Source: CAD feature listing. Evaluate the final solid. Frame: model axes, mm. Face numbers are marked on the shaded views. Give positions to 0.01 mm unless a question says otherwise; leave off trailing zeros. Write each loop counter-clockwise with the first axis right and the second up, starting at its lowest first coordinate (ties: lowest second). Pieces come first, ordered by that corner, then holes. Notation, with made-up numbers: (86, 58) -> (111, 58) arc R19 ccw to (111, 76) -> close; hole circle Ø5 at (85, 41.25). An arc over 180 degrees is marked (long way). Answer as a JSON object with one key per item and string values. Group by question number.
Item 1: Ray query, probe 1 along Z at (x, y) = (8.5, 18.5); probe 2 along X at (y, z) = (25, 232.5); probe 3 along Y at (x, z) = (-34, 32). Return the intervals inside material, ascending. Write a range as from..to.
Item 2: Section query A-A on y = 0. Return the cut outline in (x, z).
Item 3: Section query C-C on y = 13. Return the cut outline in (x, z).
Item 4: Section query D-D on z = 16.5. Return the cut outline in (x, y), plus the area to 3 significant figures.
Item 5: Section query B-B on x = 0. Return the cut outline in (y, z), plus the area to 3 significant figures.
Item 6: Pull-direction query (Y, two-part tool) for the marked faces 1, 2, 3 and 4; classes: pulls with the +Y half, pulls with the -Y half, needs draft (parallel to the pull), parting line crosses it, or undercut.
Item 7: First-contact query: pin 1 Ø10 at (x, z) = (30, 86.5) entering from -Y; pin 2 Ø5 at (y, z) = (-1, 162.5) entering from -X; pin 3 Ø3 at (x, z) = (-19, 105.5) entering from +Y. Flat tips, straight axial feed; report the tip coordinate or a pass-through.
from build123d import *

# Parameters (mm, degrees)
F0_R          = 50
F1_DEPTH      = 250
F2_W          = 50
F2_H          = 26.758289
F3_DEPTH      = 50
F3_DEPTH_BACK = 50


with BuildPart() as f1:
    # F0 (on Top) → F1 (new body)
    with BuildSketch(Plane.XY):
        Circle(F0_R)
    extrude(amount=F1_DEPTH)

    # F2 (on Right) → F3 (cut, two sides)
    with BuildSketch(Plane.YZ) as f3_sk:
        with Locations((0, 43.379144)):
            Rectangle(F2_W, F2_H)
    extrude(amount=F3_DEPTH, mode=Mode.SUBTRACT)
    extrude(f3_sk.sketch, amount=-F3_DEPTH_BACK, mode=Mode.SUBTRACT)


solid = f1.part
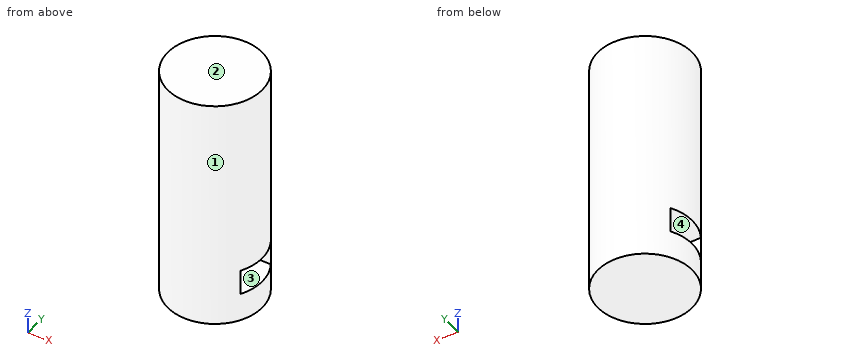
Worked answers:
{
 "1": {"probe 1": "0..30, 56.76..250", "probe 2": "-43.3..43.3", "probe 3": "-36.66..-25, 25..36.66"},
 "2": {"outline": "(-50, 0) -> (50, 0) -> (50, 30) -> (-50, 30) -> close; (-50, 56.76) -> (50, 56.76) -> (50, 250) -> (-50, 250) -> close"},
 "3": {"outline": "(-48.28, 0) -> (48.28, 0) -> (48.28, 30) -> (-48.28, 30) -> close; (-48.28, 56.76) -> (48.28, 56.76) -> (48.28, 250) -> (-48.28, 250) -> close"},
 "4": {"outline": "circle Ø100 at (0, 0)", "area": "7,850 mm^2"},
 "5": {"outline": "(-50, 0) -> (50, 0) -> (50, 250) -> (-50, 250) -> close; hole (-25, 30) -> (25, 30) -> (25, 56.76) -> (-25, 56.76) -> close", "area": "23,700 mm^2"},
 "6": {"face 1": "parting line crosses it", "face 2": "needs draft", "face 3": "undercut", "face 4": "undercut"},
 "7": {"pin 1": "y = -43.3", "pin 2": "x = -50", "pin 3": "y = 46.84"}
}
